from build123d import *

# Parameters (mm, degrees)
SKETCH_1_W          = 54
SKETCH_1_H          = 35
EXTRUDE_1_DEPTH     = 1
CUT_EXTRUDE_1_DEPTH = 1
SKETCH_3_R          = 1.6
CUT_EXTRUDE_2_DEPTH = 1


with BuildPart() as part:
    # Эскиз1 → Бобышка-Вытянуть1 (new body)
    with BuildSketch(Plane(origin=(0, 0, 0), x_dir=(1, 0, 0), z_dir=(0, 1, 0))):
        Rectangle(SKETCH_1_W, SKETCH_1_H)
    extrude(amount=EXTRUDE_1_DEPTH)

    # Эскиз2 → Вырез-Вытянуть1 (cut)
    with BuildSketch(Plane(origin=(0, 1, 0), x_dir=(1, 0, 0), z_dir=(0, 1, 0))):
        Polygon((2, 17.5), (8, 11.5), (22, 11.5), (27, 6.5), (27, 17.5), align=None)
    extrude(amount=-CUT_EXTRUDE_1_DEPTH, mode=Mode.SUBTRACT)

    # Эскиз3 → Вырез-Вытянуть2 (cut)
    with BuildSketch(Plane(origin=(0, 1, 0), x_dir=(1, 0, 0), z_dir=(0, 1, 0))):
        with Locations((-23.9, 14.5)):
            Circle(SKETCH_3_R)
        with Locations((-23.9, -14.5)):
            Circle(SKETCH_3_R)
        with Locations((23.9, -14.5)):
            Circle(SKETCH_3_R)
    extrude(amount=-CUT_EXTRUDE_2_DEPTH, mode=Mode.SUBTRACT)


solid = part.part
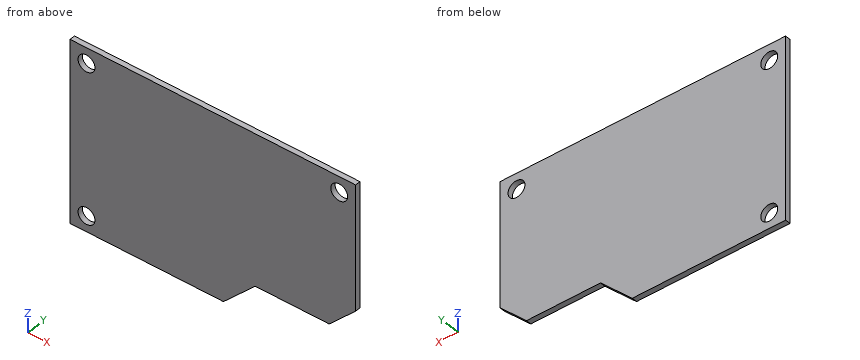
Could you check a few things on this model? Use its own coordinates, in mm. Give positions to 0.01 mm unless a question says otherwise; leave off trailing zeros. Loops run counter-clockwise (first coordinate to the right, second up) from the corner with the lowest first, then second, coordinate; pieces in that order, holes last. Notation, with made-up numbers: M 6.5,-10.75 L 35.5,-10.75 A13 cw 35.5,7.25 Z; hole C 12,21.5 d6. An arc over 180 degrees is marked long. Answer as a JSON object with one key per item and string values.
Q1. Suppose I cut it at A-A, the plane x = 23.9. List the corners of the cut face in (y, z) for me, plus the area to 3 significant figures.
Values found:
{"outline": "M 0,-9.6 L 1,-9.6 L 1,12.9 L 0,12.9 Z; M 0,16.1 L 1,16.1 L 1,17.5 L 0,17.5 Z", "area": "23.9 mm²"}
Q2. Suppose I cut it at B-B, the plane z = 14.5. List the corners of the cut face in (x, y) for me, plus the area to 3 significant figures.
Values found:
{"outline": "M -27,0 L -25.5,0 L -25.5,1 L -27,1 Z; M -22.3,0 L 22.3,0 L 22.3,1 L -22.3,1 Z; M 25.5,0 L 27,0 L 27,1 L 25.5,1 Z", "area": "47.6 mm²"}
Q3. If I drill on probe 1 along X at (y, z) = (0.45, 14.5); probe 2 along Z at (x, y) = (-23.9, 0.4); probe 3 along X at (y, z) = (0.65, -14.5), over which ranges is the centre line in solid material (lowest first)? Write a range as [from, to].
Values found:
{"probe 1": "x = [-27, -25.5], [-22.3, 22.3], [25.5, 27]", "probe 2": "z = [-17.5, -16.1], [-12.9, 12.9], [16.1, 17.5]", "probe 3": "x = [-27, -25.5], [-22.3, 5]"}
Q4. Suppose I cut it at C-C, the plane x = -23.9. List the corners of the cut face in (y, z) for me.
Values found:
{"outline": "M 0,-17.5 L 1,-17.5 L 1,-16.1 L 0,-16.1 Z; M 0,-12.9 L 1,-12.9 L 1,12.9 L 0,12.9 Z; M 0,16.1 L 1,16.1 L 1,17.5 L 0,17.5 Z"}
Q5. Suppose I cut it at D-D, the plane y = 0.35. List the corners of the cut face in (x, z) for me.
Values found:
{"outline": "M -27,-17.5 L 2,-17.5 L 8,-11.5 L 22,-11.5 L 27,-6.5 L 27,17.5 L -27,17.5 Z; hole C -23.9,-14.5 d3.2; hole C -23.9,14.5 d3.2; hole C 23.9,14.5 d3.2"}
Q6. For P1, Ø2.5, axis at x = -23.9, z = -14.5, coming from the -Y side, with a flat end and sliding along its axis, tell me the tip position at first contact or that it passes through.
Values found:
{"P1": "passes through"}
